Source: CAD feature listing. Evaluate the final solid. Frame: model axes, mm. A direction names the side the tool comes from. Round coordinates to 2 decimals unless told otherwise and drop trailing zeros. Order: outer loops, then holes, each group sorted by start corner. A loop starts at its lowest first (then second) coordinate and runs counter-clockwise, first axis right, second up. Notation, with made-up numbers: (75.25, 80.5) - (117.25, 80.5) arc R30 ccw to (117.25, 102.5) - close; hole circle Ø4 at (45.5, 52). An arc over 180 degrees is marked (long way). Use one line per item in the form item = value. Start each with the question number.
Q1. Pin query (flat end, axial travel): pin 1 Ø5 at (y, z) = (1, -1.5) entering from +X; pin 2 Ø2 at (y, z) = (-1, 2) entering from -X; pin 3 Ø2 at (x, z) = (1.5, -7) entering from +Y; pin 4 Ø2 at (x, z) = (7, -9.5) entering from +Y. Return the tip coordinate at first contact, or that it passes through.
Q2. Ray query, line 1 (Z direction, x = 2.5, y = -7.75); line 2 (Z direction, x = 6.25, y = 1.75); line 3 (Y direction, x = 8.3, z = 8). Return the intervals inside material, ascending. Write a range as [from, to].
Q3. Cut plane C-C, the plane y = -7. Return the cut outline in (x, z), and give its area (3 significant figures).
Q4. Draft query along X for faces 5 (the flat face through (10, -4, -2)), 6 (the cylindrical face through (4.93, -11.664, 2.82)), 7 (the flat face through (5, -5, -6)). Return one class per face: released by +X, released by -X, zero draft, split by the parting line, or undercut.
Q5. Cut plane B-B, the plane z = 8. Return the cut outline in (x, y).
Q6. Cut plane A-A, the plane x = 5. Return the cut outline in (y, z).
Q7. Set-up query: faces 1 (the flat face through (8.044, -6.772, -6.479)), 2 (the cylindrical face through (7.972, -0.143, -4.753)), 3 (the flat face through (5, -6, -0.6)), 4 (the flat face through (5.1, -4.7, -8)). Return all of +Z, -Z, +X, -X, +Y, -Y with unobstructed straight access to the full face (end or side cutting, diameter ignored); none if empty.
Q8. Cut plane D-D, the plane z = -1.5. Return the cut outline in (x, y), and give its area (3 significant figures).
Autodesk Inventor part; units mm, degrees
ref_plane "YZ Plane" through (0, 0, 0) normal (1, 0, 0) x (0, 1, 0)
ref_plane "XZ Plane" through (0, 0, 0) normal (0, 1, 0) x (-1, 0, 0)
ref_plane "XY Plane" through (0, 0, 0) normal (0, 0, 1) x (1, 0, 0)
sketch "スケッチ1" plane through (0, 0, 0) normal (1, 0, 0) x (0, 1, 0)
  circle A0 centre (0, 0) radius 4.2
  circle A1 centre (0, 0) radius 8.5
  line L0 (0, 5) -> (-12, 5)
  line L1 (-12, 5) -> (-12, -5) construction
  line L2 (-12, -5) -> (0, -5)
  line L3 (0, -5) -> (0, 5) construction
  line L4 (-12, 0.6) -> (0, 0.6)
  line L5 (0, 0.6) -> (0, -0.6)
  line L6 (0, -0.6) -> (-12, -0.6)
  line L7 (-12, -0.6) -> (-12, 0.6)
  line L8 (4.5, 12) -> (-4.5, 12) construction
  line L9 (-4.5, 12) -> (-4.5, -12)
  line L10 (-4.5, -12) -> (4.5, -12) construction
  line L11 (4.5, -12) -> (4.5, 12)
  line L12 (4.5, 12) -> (-4.5, -12) construction
  line L13 (-4.5, 12) -> (4.5, -12) construction
  arc A2 (4.5, 11.1243) -> (-4.5, 11.1243) centre (0, 0) ccw
  arc A3 (-4.5, -11.1243) -> (4.5, -11.1243) centre (0, 0) ccw
  arc A4 (-10.9087, 5) -> (-10.9087, -5) centre (0, 0) ccw
  point P0 (-11, 3.3541)
  point P1 (-11, -3.3541)
  point P2 (-6.8739, 5)
  point P3 (-6.8739, -5)
  point P4 (-4.1569, 0.6)
  point P5 (-4.1569, -0.6)
  point P6 (-12, -0.6)
  point P7 (-8.4788, -0.6)
  point P8 (-8.4788, 0.6)
  point P9 (0, -4.2)
  point P10 (0, 4.2)
  point P11 (0, 0.6)
  point P12 (-4.5, -5)
  point P13 (4.5, -7.2111)
  point P14 (4.5, 7.2111)
  point P15 (-4.5, 5)
  point P16 (-4.5, -7.2111)
  point P17 (-4.5, 7.2111)
  point P18 (-4.5, 0.6)
  point P19 (-4.5, -0.6)
  point P20 (-11.985, 0.6)
  point P21 (-11.985, -0.6)
  dimension "d0" = 8.4
  dimension "d1" = 17
  dimension "d2" = 5
  dimension "d3" = 5
  dimension "d4" = 12
  dimension "d18" = 1.2
  dimension "d19" = 0.6
  dimension "d45" = 9
  dimension "d46" = 24
extrude "押し出し1" add sketch "スケッチ1" along normal blind 10 contours A0 L4 L9 A1 L11 L6 | L4 A1 L0 L9 | L9 L2 A1 L6 | L4 A4 L0 A1 | A1 L2 A4 L6 | L9 A2 L11 A1 | A1 L11 A3 L9 | A1 L11
sketch "スケッチ2" plane through (10, 0, 0) normal (1, 0, 0) x (0, 0, -1)
  line L0 (16.8, 0) -> (-16.8, 0)
  point P0 (0, 0)
  point P1 (-8, 0)
  point P2 (8, 0)
  dimension "d7" = 8
  dimension "d8" = 8
hole "穴1" at (10, 0, 8) at (10, 0, -8) direction (-1, 0, 0) diameter 3.4 end through all counterbore diameter 6.5 counterbore depth 4
sketch "スケッチ3" plane through (0, -4.5, 5) normal (0, 0, 1) x (1, 0, 0)
  line L0 (0, 0) -> (10, 0)
  point P0 (5, -4)
  point P1 (5, 0)
  dimension "d56" = 4
hole "穴2" at (5, -8.5, 5) direction (0, 0, -1) diameter 4.2 end through all
sketch "スケッチ7" plane through (0, -10.9087, -5) normal (0, 0, -1) x (-1, 0, 0)
  circle A0 centre (-5, 2.4087) radius 2.1
  line L0 (-7.0207, -1.0913) -> (-9.0415, 2.4087)
  line L1 (-9.0415, 2.4087) -> (-7.0207, 5.9087)
  line L2 (-7.0207, 5.9087) -> (-2.9793, 5.9087)
  line L3 (-2.9793, 5.9087) -> (-0.9585, 2.4087)
  line L4 (-0.9585, 2.4087) -> (-2.9793, -1.0913)
  line L5 (-2.9793, -1.0913) -> (-7.0207, -1.0913)
  line L6 (0, 6.4087) -> (-10, 6.4087)
  line L7 (-10, 0) -> (-10, 6.4087)
  line L8 (0, 0) -> (0, 6.4087)
  line L9 (-10, 2.4087) -> (-9.0415, 2.4087)
  line L10 (-0.9585, 2.4087) -> (0, 2.4087)
  circle A1 centre (-9.0415, 2.4087) radius 0.2
  circle A2 centre (-7.0207, -1.0913) radius 0.2
  circle A3 centre (-2.9793, -1.0913) radius 0.2
  circle A4 centre (-0.9585, 2.4087) radius 0.2
  circle A5 centre (-2.9793, 5.9087) radius 0.2
  circle A6 centre (-7.0207, 5.9087) radius 0.2
  point P0 (0, 10.9087)
  point P1 (-9.2415, 2.4087)
  point P2 (-8.9415, 2.5819)
  point P3 (-7.1207, 5.7355)
  point P4 (-6.8207, 5.9087)
  point P5 (-3.1793, 5.9087)
  point P6 (-2.8793, 5.7355)
  point P7 (-1.0585, 2.5819)
  point P8 (-0.7585, 2.4087)
  dimension "d48" = 7
  dimension "d49" = 0.4
  dimension "d52" = 360
extrude "押し出し5" add sketch "スケッチ7" along normal blind 3 contours L9 L7 L6 L8 L10 A4 L3 A5 L2 A6 L1 A1
properties part number "セットカラ―" material "ABS プラスチック"
Completed:
q1.pin_1 = 10
q1.pin_2 = through
q1.pin_3 = 6.02
q1.pin_4 = 4.5
q2.line_1 = [-5, -0.6], [0.6, 5]
q2.line_2 = [-11.87, -10.74], [-5.26, -3.82], [3.82, 5.26], [10.74, 11.87]
q2.line_3 = [-4.5, -3.25], [3.25, 4.5]
q3.outline = (0, -8) - (1.82, -8) - (1.82, -5) - (3.53, -5) - (3.53, -0.6) - (0, -0.6) - close; (0, 0.6) - (3.53, 0.6) - (3.53, 5) - (0, 5) - close; (6.47, -5) - (8.18, -5) - (8.18, -8) - (10, -8) - (10, -0.6) - (6.47, -0.6) - close; (6.47, 0.6) - (10, 0.6) - (10, 5) - (6.47, 5) - close
q3.area = 73.1 mm2
q4.face_5 = released by +X
q4.face_6 = zero draft
q4.face_7 = undercut
q5.outline = (0, -4.5) - (10, -4.5) - (10, -3.25) - (6, -3.25) - (6, -1.7) - (0, -1.7) - close; (0, 1.7) - (6, 1.7) - (6, 3.25) - (10, 3.25) - (10, 4.5) - (0, 4.5) - close
q6.outline = (-11.98, -0.6) arc R12 ccw to (-10.91, -5) - (-10.6, -5) - (-10.6, -0.6) - close; (-11.98, 0.6) - (-10.6, 0.6) - (-10.6, 5) - (-10.91, 5) arc R12 ccw to start; (-6.4, -5) - (-5, -5) - (-5, -8) - (-4.5, -8) - (-4.5, -11.12) arc R12 ccw to (4.5, -11.12) - (4.5, -7.21) arc R8.5 ccw to (4.5, 7.21) - (4.5, 11.12) arc R12 ccw to (-4.5, 11.12) - (-4.5, 5) - (-6.4, 5) - (-6.4, 0.6) - (-4.16, 0.6) arc R4.2 cw (long way) to (-4.16, -0.6) - (-6.4, -0.6) - close; hole circle Ø3.4 at (0, -8); hole circle Ø3.4 at (0, 8)
q7.face_1 = -Z, -Y
q7.face_2 = +X
q7.face_3 = +X, -X, -Y
q7.face_4 = -Z, +X, -X, -Y
q8.outline = (0, -11.91) - (10, -11.91) - (10, -3.92) - (0, -3.92) - close; (0, 3.92) - (10, 3.92) - (10, 8.37) - (0, 8.37) - close; hole circle Ø4.2 at (5, -8.5)
q8.area = 110 mm2
